Source: three-view drawing plus pictorial views. Frame: mm from the lowest corner of the part. Give positions to 0.01 mm unless a question says otherwise; leave off trailing zeros. Loops run counter-clockwise (first coordinate to the right, second up) from the corner with the lowest first, then second, coordinate; pieces in that order, holes last. Notation, with made-up numbers: (-1, -15) -> (32, -15) arc R24 ccw to (32, 6) -> close; hole circle Ø7 at (19, 67.25). An arc over 180 degrees is marked (long way). Answer as a JSON object with one key per item and string values. Group by question number.
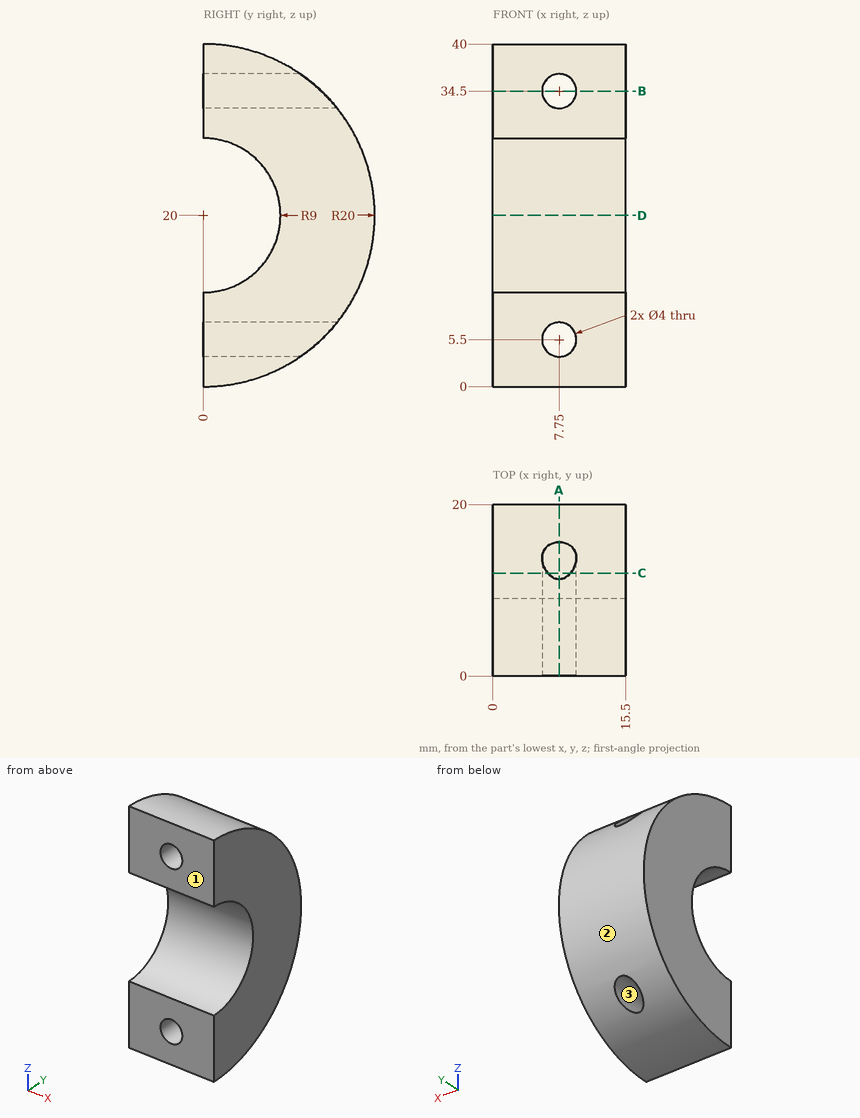
(1) Mould query, pull axis Z, two halves, no side actions, for the marked faces 1, 2 and 3. Classes: pulls with the +Z half, pulls with the -Z half, needs draft (parallel to the pull), parting line crosses it, or undercut.
(2) Section query D-D on z = 20. Return the cut outline in (x, y).
(3) Section query A-A on x = 7.75. Return the cut outline in (y, z).
(4) Section query C-C on y = 12. Return the cut outline in (x, z), plus the area to 3 significant figures.
(5) Section query B-B on z = 34.5. Return the cut outline in (x, y), plus the area to 3 significant figures.
(6) First-contact query: pin 1 (8 mm diameter, centred on x = 7, y = 6.5, fed in from +Z); pin 2 (2 mm diameter, centred on x = 7.5, y = 4.5, fed in from -Z); pin 3 (1 mm diameter, centred on x = 7.5, y = 4.5, fed in from +Z). Flat tips, straight axial feed; report the tip coordinate or a pass-through.
(7) Material intervals for line 1 (Z direction, x = 6.5, y = 4.75); line 2 (Z direction, x = 7.75, y = 4); line 3 (X direction, y = 2, z = 6), sorted ascending. Write a range as from..to.
Result:
{
 "1": {"face 1": "needs draft", "face 2": "parting line crosses it", "face 3": "undercut"},
 "2": {"outline": "(0, 9) -> (15.5, 9) -> (15.5, 20) -> (0, 20) -> close"},
 "3": {"outline": "(0, 0) arc R20 ccw to (11.3, 3.5) -> (0, 3.5) -> close; (0, 7.5) -> (15.61, 7.5) arc R20 ccw to (15.61, 32.5) -> (0, 32.5) -> (0, 29) arc R9 cw to (0, 11) -> close; (0, 36.5) -> (11.3, 36.5) arc R20 ccw to (0, 40) -> close"},
 "4": {"outline": "(0, 4) -> (6.43, 4) arc R2 cw (long way) to (9.07, 4) -> (15.5, 4) -> (15.5, 36) -> (9.07, 36) arc R2 cw (long way) to (6.43, 36) -> (0, 36) -> close", "area": "473 mm²"},
 "5": {"outline": "(0, 0) -> (5.75, 0) -> (5.75, 13.77) -> (0, 13.77) -> close; (9.75, 0) -> (15.5, 0) -> (15.5, 13.77) -> (9.75, 13.77) -> close", "area": "158 mm²"},
 "6": {"pin 1": "z = 39.84", "pin 2": "z = 0.31", "pin 3": "z = 39.6"},
 "7": {"line 1": "0.57..3.94, 7.06..12.36, 27.64..32.94, 36.06..39.43", "line 2": "0.4..3.5, 7.5..11.94, 28.06..32.5, 36.5..39.6", "line 3": "0..5.81, 9.69..15.5"}
}
